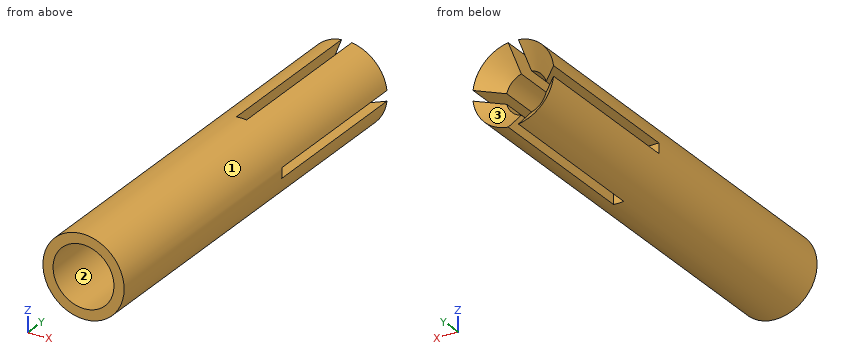
Autodesk Fusion 360 part; units mm, degrees
cylinder "CylinderPrimitive1" add diameter 2 height 10 placed x (1, 0, 0) y (0, 0, -1) z (0, 1, 0) at (0, 0, 0)
hole "Hole1" at (0, 10, 0) direction (0, -1, 0) diameter 1 depth 4 tip angle 118
hole "Hole2" at (0, 0, 0) direction (0, 1, 0) diameter 1.5 depth 4 tip angle 118
chamfer "Chamfer1" distance 0.5 angle 45 1 edges at (0.1808, 10, -0.4662) measured on face at (0.8291, 10, 0.0621)
sketch "Sketch2" plane through (0, 0, 0) normal (1, 0, 0) x (0, 0, -1)
  line L0 (-2.7313, 12.0493) -> (-0.0081, 12.0493)
  line L1 (-0.0081, 12.0493) -> (-0.0081, 6)
  line L2 (-0.0081, 6) -> (-2.7313, 6)
  line L3 (-2.7313, 6) -> (-2.7313, 12.0493)
  line L4 (1, 10) -> (-1, 10)
  dimension "d15" = 4
extrude "Extrude1" cut sketch "Sketch2" along normal mid plane 0.25
pattern_circular "C-Pattern1" count 4 over 360 about axis through (0, 1.75, 0) along (0, 1, 0) of "Extrude1"
The listing builds one solid part. Answer for the finished solid, in the listing's coordinates (mm). Face numbers are marked on the shaded views. Give positions to 0.01 mm unless a question says otherwise; leave off trailing zeros. Write each loop counter-clockwise with the first axis right and the second up, starting at its lowest first coordinate (ties: lowest second). Pieces come first, ordered by that corner, then holes. Notation, with made-up numbers: (-12.75, -25) - (-0.75, -25) arc R19 ccw to (-0.75, -12) - close; hole circle Ø11 at (-5, 63.25). An arc over 180 degrees is marked (long way). One line per question, with ' | ' between items. Start each with the question number.
1. Determine the mould class of the marked faces 1, 2 and 3 for opening direction Z: +Z half, -Z half, draft (parallel to the pull), parting line (faces both ways), or undercut.
2. Straight lines are drawn through the part: line 1 (X direction, y = 2.1, z = 0); line 2 (X direction, y = 5.25, z = 0.1). For each, find the intervals that lie inside material, in ascending order.
3. Given P1, Ø0.9, axis at x = 0, z = 0, coming from the +Y side; P2, Ø0.6, axis at x = 0.5, y = 8.5, coming from the +Z side, each flat-ended and moving along its own axis, determine where each tip first touches the part or whether it passes through.
4. Section A-A, the plane y = 6.25 is taken. Determine the outline of the cut face in (x, z) (3 decimals).
5. Section B-B, the plane y = 1.75 is taken. Determine the outline of the cut face in (x, z), then the cut area to 3 significant figures.
Result:
1) face 1: parting line | face 2: undercut | face 3: undercut
2) line 1: x = -1 to -0.75, 0.75 to 1 | line 2: x = -0.99 to 0.99
3) P1: stops at y = 5.97 | P2: stops at z = 0.98
4) outline: (-0.992, -0.125) arc R1 ccw to (-0.125, -0.992) - (-0.125, -0.484) arc R0.5 cw to (-0.484, -0.125) - close; (-0.992, 0.125) - (-0.484, 0.125) arc R0.5 cw to (-0.125, 0.484) - (-0.125, 0.992) arc R1 ccw to start; (0.125, -0.992) arc R1 ccw to (0.992, -0.125) - (0.484, -0.125) arc R0.5 cw to (0.125, -0.484) - close; (0.125, 0.484) arc R0.5 cw to (0.484, 0.125) - (0.992, 0.125) arc R1 ccw to (0.125, 0.992) - close
5) outline: circle Ø2 at (0, 0); hole circle Ø1.5 at (0, 0) | area: 1.37 mm2
